from build123d import *

# Parameters (mm, degrees)
F1_DEPTH = 36


with BuildPart() as f1:
    # F0 (on Top) → F1 (new body)
    with BuildSketch(Plane.XY):
        with BuildLine():
            Line((-288.386514, -22.46141), (-288.386514, -152.46141))
            Line((-288.386514, -152.46141), (-53.386514, -152.46141))
            Line((-53.386514, -152.46141), (-53.386514, -77.46141))
            Line((-53.386514, -77.46141), (42.613486, -77.46141))
            Line((42.613486, -77.46141), (42.613486, -152.46141))
            Line((42.613486, -152.46141), (277.613486, -152.46141))
            Line((277.613486, -152.46141), (277.613486, 117.53859))
            Line((277.613486, 117.53859), (23.203639, 117.53859))
            ThreePointArc((23.203639, 117.53859), (4.079002, 101.6535), (-1.967393, 77.53859))
            Line((-1.967393, 77.53859), (-1.967393, 17.53859))
            ThreePointArc((-1.967393, 17.53859), (-14.864905, -12.026696), (-45.386514, -22.46141))
            Line((-45.386514, -22.46141), (-288.386514, -22.46141))
        make_face()
    extrude(amount=F1_DEPTH)


solid = f1.part
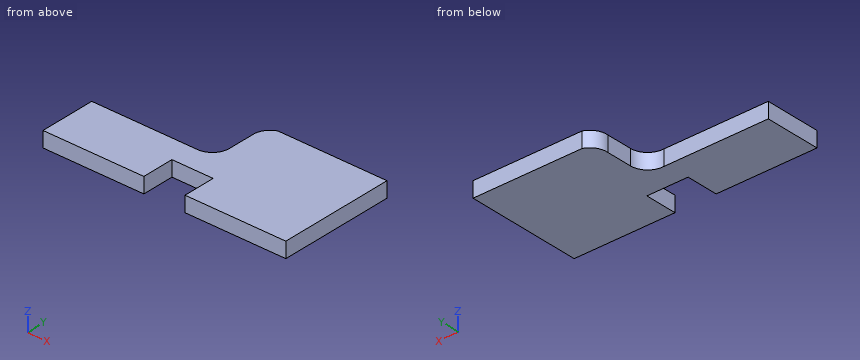
Can you work these out from the model? Positions are in its coordinate system, mm. Coordinates: 2 decimals unless noted, no trailing zeros. Order: outer loops, then holes, each group sorted by start corner. A loop starts at its lowest first (then second) coordinate and runs counter-clockwise, first axis right, second up. Notation, with made-up numbers: (87.5, -21) -> (103.5, -21) arc R20 ccw to (103.5, 18) -> close; hole circle Ø6 at (67.25, 0). An arc over 180 degrees is marked (long way). Use one line per item in the form item = value.
Q1. Imagine slicing it at B-B, the plane z = 27.5. List the corners of the cut face in (x, y) for me.
From the geometry:
outline = (-288.39, -152.46) -> (-53.39, -152.46) -> (-53.39, -77.46) -> (42.61, -77.46) -> (42.61, -152.46) -> (277.61, -152.46) -> (277.61, 117.54) -> (23.2, 117.54) arc R40 ccw to (-1.97, 77.54) -> (-1.97, 17.54) arc R40 cw to (-45.39, -22.46) -> (-288.39, -22.46) -> close
Q2. I need wall thicknesses on L1, parallel to X at y = -140, z = 15; L2, parallel to Y at x = -68, z = 4; L3, parallel to X at y = 36, z = 11.5. Which ranges of each line are inside material? Lowest first, please.
From the geometry:
L1 = -288.39 to -53.39, 42.61 to 277.61
L2 = -152.46 to -22.46
L3 = -1.97 to 277.61
Q3. Will these pins go through, and if not, where does the flat tip stop? P1, Ø5, axis at x = -167, z = 5.5, coming from the +Y side; P2, Ø12, axis at y = 9.5, z = 8, coming from the -X side.
From the geometry:
P1 = -22.46
P2 = -4.46
Q4. Imagine slicing it at D-D, the plane x = -78.5. List the corners of the cut face in (y, z) for me.
From the geometry:
outline = (-152.46, 0) -> (-22.46, 0) -> (-22.46, 36) -> (-152.46, 36) -> close
Q5. Imagine slicing it at A-A, the plane y = -105. List the corners of the cut face in (x, z) for me, then the cut area to 3 significant figures.
From the geometry:
outline = (-288.39, 0) -> (-53.39, 0) -> (-53.39, 36) -> (-288.39, 36) -> close; (42.61, 0) -> (277.61, 0) -> (277.61, 36) -> (42.61, 36) -> close
area = 16,900 mm²
Q6. Imagine slicing it at C-C, the plane y = 32.5. List the corners of the cut face in (x, z) for me, then the cut area to 3 significant figures.
From the geometry:
outline = (-1.97, 0) -> (277.61, 0) -> (277.61, 36) -> (-1.97, 36) -> close
area = 10,100 mm²
